from build123d import *

# Parameters (mm, degrees)
SKETCH1_W                       = 48
SKETCH1_H                       = 30
SKETCH1_R                       = 2.2
BOSS_EXTRUDE1_DEPTH             = 10
BOSS_EXTRUDE2_REACH             = 41.699
SKETCH3_W                       = 20
SKETCH3_H                       = 20
BOSS_EXTRUDE2_DIRECTION_2_DEPTH = 15
CUT_EXTRUDE1_START              = -30
CUT_EXTRUDE1_DEPTH              = 30
SKETCH5_R                       = 3.2639
CUT_EXTRUDE2_DEPTH              = 44.312815655
FILLET2_R                       = 2


with BuildPart() as part:
    # Sketch1 → Boss-Extrude1 (new body)
    with BuildSketch(Plane(origin=(0, 0, 0), x_dir=(1, 0, 0), z_dir=(0, 1, 0))):
        Rectangle(SKETCH1_W, SKETCH1_H)
        with Locations(Location((-20, 10, 0), (0, 0, 270))):
            Circle(SKETCH1_R, mode=Mode.SUBTRACT)
        with Locations(Location((20, 10, 0), (0, 0, 270))):
            Circle(SKETCH1_R, mode=Mode.SUBTRACT)
        with Locations(Location((20, -10, 0), (0, 0, 270))):
            Circle(SKETCH1_R, mode=Mode.SUBTRACT)
        with Locations(Location((-20, -10, 0), (0, 0, 270))):
            Circle(SKETCH1_R, mode=Mode.SUBTRACT)
    extrude(amount=BOSS_EXTRUDE1_DEPTH)

    # Boss-Extrude2: up to this face of the body (flat: up to its plane)
    boss_extrude2_end = Plane(part.part.faces().sort_by_distance((0, 5, 15))[0])
    # Sketch3 → Boss-Extrude2 (add, up to the picked face)
    with BuildSketch(Plane(origin=(0, 0, -15), x_dir=(-1, 0, 0), z_dir=(0, 0, -1)), mode=Mode.PRIVATE) as boss_extrude2_sk1:
        with Locations((0, 10)):
            Rectangle(SKETCH3_W, SKETCH3_H)
    boss_extrude2_tool1 = split(extrude(boss_extrude2_sk1.sketch, amount=-BOSS_EXTRUDE2_REACH, mode=Mode.PRIVATE), bisect_by=boss_extrude2_end, keep=Keep.BOTH, mode=Mode.PRIVATE)
    add(boss_extrude2_tool1.solids().sort_by(Axis((0, 10, -15), (0, 0, 1)))[0])

    # Sketch3 → Boss-Extrude2 direction 2 (add)
    with BuildSketch(Plane(origin=(0, 0, -15), x_dir=(-1, 0, 0), z_dir=(0, 0, -1))):
        with Locations((0, 10)):
            Rectangle(SKETCH3_W, SKETCH3_H)
    extrude(amount=BOSS_EXTRUDE2_DIRECTION_2_DEPTH)

    # Sketch4 → Cut-Extrude1 (cut)
    with BuildSketch(Plane(origin=(0, 0, -30), x_dir=(-1, 0, 0), z_dir=(0, 0, -1)).offset(CUT_EXTRUDE1_START)):
        Polygon((-6.5, 13.75277675), (-6.5, 6.24722325), (0, 2.494446501), (6.5, 6.24722325), (6.5, 13.75277675), (0, 17.505553499), align=None)
    extrude(amount=CUT_EXTRUDE1_DEPTH, mode=Mode.SUBTRACT)

    # Sketch5 → Cut-Extrude2 (cut, through all)
    with BuildSketch(Plane(origin=(0, 0, -15), x_dir=(-1, 0, 0), z_dir=(0, 0, -1))):
        with Locations((0, 10)):
            Circle(SKETCH5_R)
    extrude(amount=-CUT_EXTRUDE2_DEPTH, mode=Mode.SUBTRACT)

    # Fillet2
    fillet2_edges = [part.edges().sort_by_distance(p)[0] for p in [
        (-10, 5, -15),
        (10, 5, -15),
        (10, 10, 0),
        (10, 20, -7.5),
        (-10, 10, 0),
        (-10, 20, -7.5),
        (-24, 5, -15),
        (24, 5, -15),
        (24, 5, 15),
        (-24, 5, 15),
    ]]
    fillet(fillet2_edges, radius=FILLET2_R)


solid = part.part
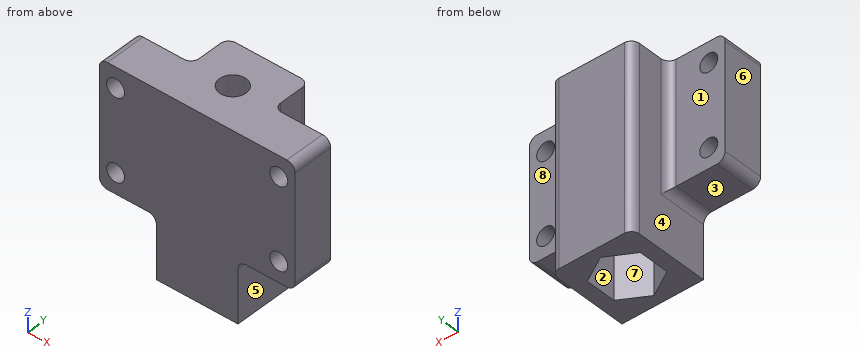
For this review, take the finished solid that the model builds, in its own axes (mm). Face numbers are marked on the shaded views. A direction names the side the tool comes from. Round coordinates to 2 decimals unless told otherwise and drop trailing zeros. Loops run counter-clockwise (first coordinate to the right, second up) from the corner with the lowest first, then second, coordinate; pieces in that order, holes last. Notation, with made-up numbers: (48.25, -16.5) - (76.25, -16.5) arc R13 cw to (76.25, -2.5) - close; hole circle Ø7 at (-11.75, -6.5). An arc over 180 degrees is marked (long way). Use one line per item in the form item = value.
Item 1: Consider section D-D on z = -24. Write out the cut boundary in (x, y).
Answers:
outline = (-10, 0) - (10, 0) - (10, 18) arc R2 ccw to (8, 20) - (-8, 20) arc R2 ccw to (-10, 18) - close; hole (-6.5, 6.25) - (0, 2.49) - (6.5, 6.25) - (6.5, 13.75) - (0, 17.51) - (-6.5, 13.75) - close
Item 2: Mouldability with a two-part tool opening along Y and no side actions: class the marked faces 6, 7 and 8 as +Y half, -Y half, draft (parallel to the pull), parting line (faces both ways), or undercut.
Answers:
face_6 = draft
face_7 = undercut
face_8 = +Y half
Item 3: Clearance check with flat-ended pins moving along their axes: P1, Ø9.5, axis at x = -17, z = -3, coming from the +Y side; P2, Ø1, axis at y = 6, z = -16.5, coming from the +X side; P3, Ø4, axis at x = -20, z = 10, coming from the +Y side; P4, Ø8.5, axis at x = 0, y = 10, coming from the -Z side. State where each tip first meets the part, or that it passes through.
Answers:
P1 = 10
P2 = 10.27
P3 = through
P4 = 0
Item 4: Consider section C-C on x = -1. Write out the cut boundary in (y, z).
Answers:
outline = (0, -30) - (3.07, -30) - (3.07, 0) - (6.89, 0) - (6.89, 15) - (0, 15) - close; (13.11, 0) - (16.93, 0) - (16.93, -30) - (20, -30) - (20, 15) - (13.11, 15) - close
Item 5: Tool access review of the marked faces 1, 2, 3, 4 and 5: name each direction out of +Z, -Z, +X, -X, +Y, -Y from which nothing blocks a thin tool from reaching the whole face with its end or side.
Answers:
face_1 = +Z, -Z, -X, +Y
face_2 = -Z
face_3 = -Z, -X, +Y, -Y
face_4 = -Z, -X, +Y
face_5 = -Z, +X, +Y
Item 6: For line 1 (X direction, y = 5, z = 10); line 2 (X direction, y = 6.5, z = -10); line 3 (X direction, y = 8.5, z = -13), list the stretches that pass through material, from the lowest coordinate up.
Answers:
line_1 = -24 to -22.2, -17.8 to 17.8, 22.2 to 24
line_2 = -24 to -22.2, -17.8 to -6.5, 6.5 to 17.8, 22.2 to 24
line_3 = -24 to -6.5, 6.5 to 24
Item 7: Consider section B-B on x = 20. Write out the cut boundary in (y, z), then the cut area to 3 significant figures.
Answers:
outline = (0, -15) - (10, -15) - (10, -12.2) - (0, -12.2) - close; (0, -7.8) - (10, -7.8) - (10, 7.8) - (0, 7.8) - close; (0, 12.2) - (10, 12.2) - (10, 15) - (0, 15) - close
area = 212 mm^2
Item 8: Consider section A-A on z = -10. Write out the cut boundary in (x, y), then the cut area to 3 significant figures.
Answers:
outline = (-24, 0) - (-22.2, 0) - (-22.2, 10) - (-24, 10) - close; (-17.8, 0) - (17.8, 0) - (17.8, 10) - (12, 10) arc R2 cw to (10, 12) - (10, 18) arc R2 ccw to (8, 20) - (-8, 20) arc R2 ccw to (-10, 18) - (-10, 12) arc R2 cw to (-12, 10) - (-17.8, 10) - close; (22.2, 0) - (24, 0) - (24, 10) - (22.2, 10) - close; hole (-6.5, 6.25) - (0, 2.49) - (6.5, 6.25) - (6.5, 13.75) - (0, 17.51) - (-6.5, 13.75) - close
area = 446 mm^2
